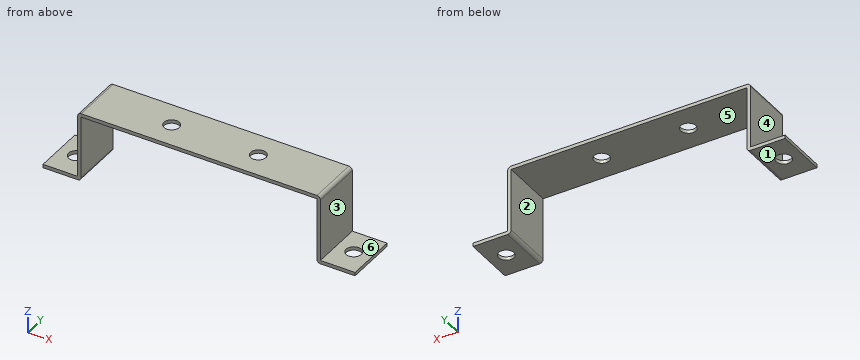
```python
from build123d import *

# Parameters (mm, degrees)
F1_DEPTH = 30
F2_R     = 4.4
F3_R     = 4.4
F4_DEPTH = 25
F5_R     = 2
F6_R     = 2


# Not quite as in the source:
# - a feature names something its author has since deleted; it is built from what else it names


with BuildPart() as f1:
    # F0 (on Front) → F1 (new body)
    with BuildSketch(Plane.XZ):
        Polygon((90, -1), (90, 1), (70, 1), (70, 39), (-70, 39), (-70, 1), (-90, 1), (-90, -1), (-68, -1), (-68, 37), (68, 37), (68, -1), align=None)
    extrude(amount=F1_DEPTH)

    # F2 (on face) + F3 (on face) → F4 (cut)
    with BuildSketch(Plane.XY.offset(1)):
        with Locations((-80, -15)):
            Circle(F2_R)
        with Locations((80, -15)):
            Circle(F2_R)
    with BuildSketch(Plane.XY.offset(39)):
        with Locations((-25, -15)):
            Circle(F3_R)
        with Locations((25, -15)):
            Circle(F3_R)
    extrude(amount=-F4_DEPTH, mode=Mode.SUBTRACT)

    # F5
    f5_edges = [f1.edges().sort_by_distance(p)[0] for p in [
        (-70, -15, 39),
        (70, -15, 39),
    ]]
    fillet(f5_edges, radius=F5_R)

    # F6
    f6_edges = [f1.edges().sort_by_distance(p)[0] for p in [
        (68, -15, -1),
        (-68, -15, -1),
    ]]
    fillet(f6_edges, radius=F6_R)


solid = f1.part
```
The model under review builds one solid part; all positions refer to its coordinate system, in mm. Face numbers are marked on the shaded views. A direction names the side the tool comes from. Round coordinates to 2 decimals unless told otherwise and drop trailing zeros. Write each loop counter-clockwise with the first axis right and the second up, starting at its lowest first coordinate (ties: lowest second). Pieces come first, ordered by that corner, then holes. Notation, with made-up numbers: M 16,-24 L 72,-24 A18 cw 72,11 Z; hole C 44,70.5 d1. An arc over 180 degrees is marked long. Use CSV: the item, a comma, the result in double quotes. Start each with the question number.
(1) For line 1 along Y through (x, z) = (-25, 38); line 2 along X through (y, z) = (-2.5, 33.5); line 3 along Z through (x, y) = (61, -8.5), list the stretches that pass through material, from the lowest coordinate up.
(2) We need section C-C, the plane y = -13. State how many separate pieces and enclosed holes the cut face has, then the cut area to 3 significant figures.
(3) We need section B-B, the plane z = 20. State the section outline as (x, y) points, then the cut area to 3 significant figures.
(4) We need section A-A, the plane x = -25. State the section outline as (y, z) points, then the cut area to 3 significant figures.
(5) Clearance check with flat-ended pins moving along their axes: P1, Ø16, axis at x = -80.5, y = -12.5, coming from the +Z side; P2, Ø15, axis at y = -15, z = 13, coming from the +X side; P3, Ø12, axis at y = -9, z = 14, coming from the -X side. State where each tip first meets the part, or that it passes through.
(6) The part is to be moulded in two halves that separate along X. For the marked faces 1, 2 and 3, say which applies: +X half, -X half, draft (parallel to the pull), parting line (faces both ways), or undercut.
(7) Tool access review of the marked faces 4, 5 and 6: name each direction out of +Z, -Z, +X, -X, +Y, -Y from which nothing blocks a thin tool from reaching the whole face with its end or side.
(8) We need section D-D, the plane x = -63.5. State the section outline as (y, z) points.
Findings:
1,line 1,"-30 to -19.4, -10.6 to 0"
1,line 2,"-70 to -68, 68 to 70"
1,line 3,"37 to 39"
2,separate pieces,"5"
2,enclosed holes,"0"
2,area,"446 mm^2"
3,outline,"M -70,-30 L -68,-30 L -68,0 L -70,0 Z; M 68,-30 L 70,-30 L 70,0 L 68,0 Z"
3,area,"120 mm^2"
4,outline,"M -30,37 L -19.4,37 L -19.4,39 L -30,39 Z; M -10.6,37 L 0,37 L 0,39 L -10.6,39 Z"
4,area,"42.4 mm^2"
5,P1,"z = 1"
5,P2,"x = 70"
5,P3,"x = -70"
6,face 1,"draft"
6,face 2,"undercut"
6,face 3,"+X half"
7,face 4,"+Z, -X, +Y, -Y"
7,face 5,"-Z, +Y, -Y"
7,face 6,"+Z, +X, +Y, -Y"
8,outline,"M -30,37 L 0,37 L 0,39 L -30,39 Z"
